Geometry: final body of the model. Coordinates: model frame, mm. A direction names the side the tool comes from. Round coordinates to 2 decimals unless told otherwise and drop trailing zeros. Order: outer loops, then holes, each group sorted by start corner. A loop starts at its lowest first (then second) coordinate and runs counter-clockwise, first axis right, second up. Notation, with made-up numbers: M -14.5,2.5 L 44.5,2.5 A23 ccw 44.5,16.5 Z; hole C 72,88 d9. An arc over 180 degrees is marked long. Put each result on its own line as item: value. Start each with the question number.
1) Draft query along X for faces 1 (the flat face through (0, 10, -3)), 2 (the flat face through (-13.029, -0.036, 4.322)), 3 (the cylindrical face through (-16.814, -0.846, 1.52)), 4 (the flat face through (-7, 0, -6.35)). Return one class per face: pulls with the +X half, pulls with the -X half, needs draft (parallel to the pull), parting line crosses it, or undercut.
2) Section C-C, the plane z = -4.5. Return loops of the section in (x, y), then the cut area to 3 significant figures.
3) First-contact query: P1, Ø1, axis at x = -4.5, z = 4, coming from the -Y side; P2, Ø1, axis at y = 3, z = -4.5, coming from the -X side; P3, Ø3, axis at x = -16, z = -3, coming from the -Y side. Flat tips, straight axial feed; report the tip coordinate or a pass-through.
4) Section A-A, the plane y = 11.25. Return loops of the section in (x, z).
5) Section D-D, the plane z = -1. Return loops of the section in (x, y).
6) Material intervals for probe 1 along X at (y, z) = (22, 2.25); probe 2 along Z at (x, y) = (-0.75, 11.5); probe 3 along Y at (x, z) = (-1.25, -5.5), sorted ascending. Write a range as [from, to].
7) Section B-B, the plane z = 3. Return loops of the section in (x, y), then the cut area to 3 significant figures.
8) Access query for faces 5 (the flat face through (-1, 16, -3)), 6 (the flat face through (-7, 0, 6.35)). Directions: +Z, -Z, +X, -X, +Y, -Y. A direction counts if a zero-diameter tool reaches every point of the face in a straight line with its end or side. Return the directions, or none.
from build123d import *

# Parameters (mm, degrees)
BOSS_EXTRUDE1_DEPTH            = 6.35
F_5_16_0_3125_DIAMETER_HOLE1_D = 7.9375
F_5_16_0_3125_DIAMETER_HOLE2_D = 7.9375


with BuildPart() as part:
    # Sketch1 → Boss-Extrude1 (new body, symmetric)
    with BuildSketch(Plane.XY):
        Polygon((0, 0), (0, 25.4), (-1, 25.4), (-1, 0.923419949), (-25.399102496, -1.022542132), (-25.319599474, -2.019376756), align=None)
    extrude(amount=BOSS_EXTRUDE1_DEPTH, both=True)

    # 5/16 (0.3125) Diameter Hole1 (through all)
    with Locations(Plane(origin=(-1, 13.161709974, 0), x_dir=(0, -1, 0), z_dir=(-1, 0, 0))):
        with Locations((0, 0)):
            Hole(F_5_16_0_3125_DIAMETER_HOLE1_D / 2)

    # 5/16 (0.3125) Diameter Hole2 (through all)
    with Locations(Plane(origin=(-13.199551248, -0.049561091, 0), x_dir=(0.996834625, 0.079503022, 0), z_dir=(-0.079503022, 0.996834625, 0))):
        with Locations((0, 0)):
            Hole(F_5_16_0_3125_DIAMETER_HOLE2_D / 2)


solid = part.part
Result sheet:
1. face 1: pulls with the +X half
1. face 2: pulls with the -X half
1. face 3: undercut
1. face 4: needs draft
2. outline: M -25.4,-1.02 L -25.32,-2.02 L 0,0 L 0,25.4 L -1,25.4 L -1,0.92 Z
2. area: 49.9 mm2
3. P1: stops at y = -0.4
3. P2: stops at x = -1
3. P3: stops at y = -1.4
4. outline: M -1,-6.35 L 0,-6.35 L 0,-3.48 L -1,-3.48 Z; M -1,3.48 L 0,3.48 L 0,6.35 L -1,6.35 Z
5. outline: M -25.4,-1.02 L -25.32,-2.02 L -16.95,-1.35 L -17.03,-0.35 Z; M -9.37,0.26 L -9.29,-0.74 L 0,0 L 0,9.32 L -1,9.32 L -1,0.92 Z; M -1,17 L 0,17 L 0,25.4 L -1,25.4 Z
6. probe 1: x = [-1, 0]
6. probe 2: z = [-6.35, -3.6], [3.6, 6.35]
6. probe 3: y = [-0.1, 0.9]
7. outline: M -25.4,-1.02 L -25.32,-2.02 L -15.71,-1.25 L -15.79,-0.26 Z; M -10.61,0.16 L -10.53,-0.84 L 0,0 L 0,10.56 L -1,10.56 L -1,0.92 Z; M -1,15.76 L 0,15.76 L 0,25.4 L -1,25.4 Z
7. area: 39.5 mm2
8. face 5: +Z, -Z, -X, +Y
8. face 6: +Z, +X, -X, +Y, -Y
